Geometry: see drawing. Coordinates: mm, zero at the bounding-box minimum. Give positions to 0.01 mm unless a question says otherwise; leave off trailing zeros. Order: outer loops, then holes, each group sorted by start corner. A loop starts at its lowest first (then second) coordinate and runs counter-clockwise, first axis right, second up. Notation, with made-up numbers: (17.5, -10) - (63.5, -10) arc R7 ccw to (63.5, -3) - close; hole circle Ø8 at (-19, 25). An arc over 180 degrees is marked (long way). Put each result on its own line as item: value. Start each with the question number.
1. Section A-A on z = 102.5. Return the cut outline in (x, y).
2. Section B-B on x = 15. Return the cut outline in (y, z).
3. Ray query, line 1 along X through (y, z) = (235, 44.5); line 2 along Y through (x, z) = (54, 29.5); line 3 along Y through (x, z) = (29.5, 115) (1 decimal). Return the intervals inside material, ascending. Write a range as from..to.
4. First-contact query: P1, Ø6, axis at x = 56, y = 275.5, coming from the -Z side; P2, Ø2, axis at x = 16.5, z = 23, coming from the +Y side; P3, Ø1.5, axis at x = 79.5, z = 77, coming from the +Y side. Flat tips, straight axial feed; report the tip coordinate or a pass-through.
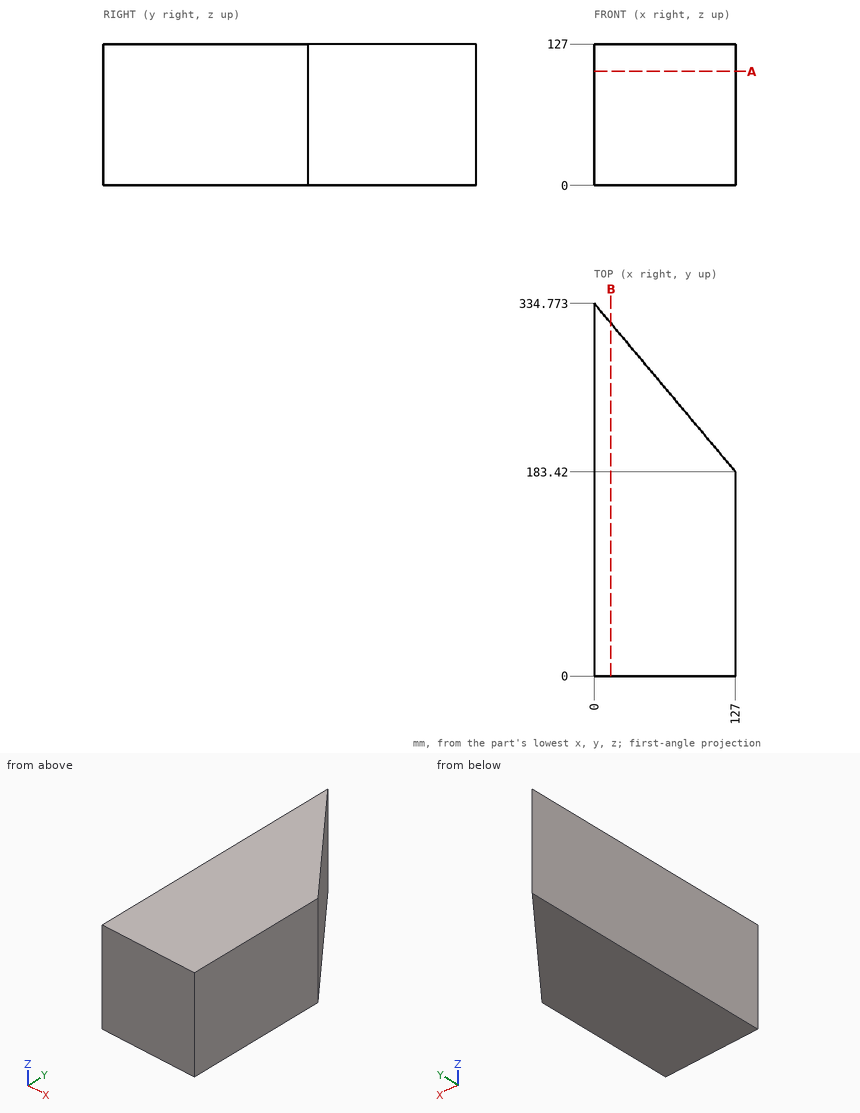
Resolved:
1. outline: (0, 0) - (127, 0) - (127, 183.42) - (0, 334.77) - close
2. outline: (0, 0) - (316.9, 0) - (316.9, 127) - (0, 127) - close
3. line 1: 0..83.72
3. line 2: 0..270.42
3. line 3: 0..299.6
4. P1: through
4. P2: y = 316.3
4. P3: y = 240.92
